Build history of the part. All positions in model axes, mm. A direction names the side the tool comes from. Round coordinates to 2 decimals unless told otherwise and drop trailing zeros. Loops run counter-clockwise (first coordinate to the right, second up) from the corner with the lowest first, then second, coordinate; pieces in that order, holes last. Notation, with made-up numbers: M 57,87 L 85,87 A16 cw 85,110 Z; hole C 41.25,71 d3. An arc over 180 degrees is marked long. One line per item, written item: value.
```python
from build123d import *

# Parameters (mm, degrees)
SKETCH1_W           = 85.598
SKETCH1_H           = 85.598
BOSS_EXTRUDE1_DEPTH = 66.04
CUT_EXTRUDE1_DEPTH  = 55.88
CUT_EXTRUDE2_DEPTH  = 55.88
CUT_EXTRUDE3_DEPTH  = 55.88
CUT_EXTRUDE4_DEPTH  = 55.88
CUT_EXTRUDE5_DEPTH  = 55.88
CUT_EXTRUDE6_DEPTH  = 55.88
CUT_EXTRUDE7_DEPTH  = 55.88
CUT_EXTRUDE8_DEPTH  = 55.88
SKETCH10_R          = 36.5125
BOSS_EXTRUDE2_DEPTH = 1.524
SKETCH11_R          = 6.35
BOSS_EXTRUDE3_DEPTH = 35.56
CUT_EXTRUDE9_DEPTH  = 25.4
CUT_EXTRUDE10_DEPTH = 25.4
SKETCH14_W          = 0.635
SKETCH14_H          = 71.501
SKETCH15_W          = 0.635
SKETCH15_H          = 71.501
SKETCH16_W          = 0.635
SKETCH16_H          = 71.501
SKETCH17_W          = 0.635
SKETCH17_H          = 71.501
HOLE1_D             = 6.604
HOLE1_DEPTH         = 47.244
HOLE2_D             = 6.604
HOLE2_DEPTH         = 47.244
HOLE3_D             = 6.604
HOLE3_DEPTH         = 47.244
HOLE4_D             = 6.604
HOLE4_DEPTH         = 47.244
CHAMFER1_SIZE       = 0.254
CHAMFER2_SIZE       = 0.254
FILLET1_R           = 2.54
FILLET2_R           = 2.54
FILLET3_R           = 2.54
FILLET4_R           = 2.54
FILLET5_R           = 2.54
FILLET6_R           = 2.54
FILLET7_R           = 2.54
FILLET8_R           = 2.54


with BuildPart() as part:
    # Sketch1 → Boss-Extrude1 (new body)
    with BuildSketch(Plane.XY.offset(66.04)):
        Rectangle(SKETCH1_W, SKETCH1_H)
    extrude(amount=-BOSS_EXTRUDE1_DEPTH)

    # Sketch2 → Cut-Extrude1 (cut)
    with BuildSketch(Plane(origin=(0, 0, 0), x_dir=(-1, 0, 0), z_dir=(0, 0, -1))):
        with BuildLine():
            Line((-42.799, -42.799), (-24.420683344, -42.799))
            ThreePointArc((-24.420683344, -42.799), (-34.84339375, -34.84339375), (-42.799, -24.420683344))
            Line((-42.799, -24.420683344), (-42.799, -42.799))
        make_face()
    extrude(amount=-CUT_EXTRUDE1_DEPTH, mode=Mode.SUBTRACT)

    # Sketch3 → Cut-Extrude2 (cut)
    with BuildSketch(Plane(origin=(0, 0, 0), x_dir=(-1, 0, 0), z_dir=(0, 0, -1))):
        with BuildLine():
            Line((-28.2194, -40.395416072), (-28.2194, -28.2194))
            Line((-28.2194, -28.2194), (-40.395416072, -28.2194))
            ThreePointArc((-40.395416072, -28.2194), (-34.84339375, -34.84339375), (-28.2194, -40.395416072))
        make_face()
    extrude(amount=-CUT_EXTRUDE2_DEPTH, mode=Mode.SUBTRACT)

    # Sketch4 → Cut-Extrude3 (cut)
    with BuildSketch(Plane(origin=(0, 0, 0), x_dir=(-1, 0, 0), z_dir=(0, 0, -1))):
        with BuildLine():
            Line((-42.799, 42.799), (-42.799, 24.420683344))
            ThreePointArc((-42.799, 24.420683344), (-34.84339375, 34.84339375), (-24.420683344, 42.799))
            Line((-24.420683344, 42.799), (-42.799, 42.799))
        make_face()
    extrude(amount=-CUT_EXTRUDE3_DEPTH, mode=Mode.SUBTRACT)

    # Sketch5 → Cut-Extrude4 (cut)
    with BuildSketch(Plane(origin=(0, 0, 0), x_dir=(-1, 0, 0), z_dir=(0, 0, -1))):
        with BuildLine():
            Line((-40.395416072, 28.2194), (-28.2194, 28.2194))
            Line((-28.2194, 28.2194), (-28.2194, 40.395416072))
            ThreePointArc((-28.2194, 40.395416072), (-34.84339375, 34.84339375), (-40.395416072, 28.2194))
        make_face()
    extrude(amount=-CUT_EXTRUDE4_DEPTH, mode=Mode.SUBTRACT)

    # Sketch6 → Cut-Extrude5 (cut)
    with BuildSketch(Plane(origin=(0, 0, 0), x_dir=(-1, 0, 0), z_dir=(0, 0, -1))):
        with BuildLine():
            Line((42.799, 42.799), (24.420683344, 42.799))
            ThreePointArc((24.420683344, 42.799), (34.84339375, 34.84339375), (42.799, 24.420683344))
            Line((42.799, 24.420683344), (42.799, 42.799))
        make_face()
    extrude(amount=-CUT_EXTRUDE5_DEPTH, mode=Mode.SUBTRACT)

    # Sketch7 → Cut-Extrude6 (cut)
    with BuildSketch(Plane(origin=(0, 0, 0), x_dir=(-1, 0, 0), z_dir=(0, 0, -1))):
        with BuildLine():
            Line((28.2194, 40.395416072), (28.2194, 28.2194))
            Line((28.2194, 28.2194), (40.395416072, 28.2194))
            ThreePointArc((40.395416072, 28.2194), (34.84339375, 34.84339375), (28.2194, 40.395416072))
        make_face()
    extrude(amount=-CUT_EXTRUDE6_DEPTH, mode=Mode.SUBTRACT)

    # Sketch8 → Cut-Extrude7 (cut)
    with BuildSketch(Plane(origin=(0, 0, 0), x_dir=(-1, 0, 0), z_dir=(0, 0, -1))):
        with BuildLine():
            Line((42.799, -42.799), (42.799, -24.420683344))
            ThreePointArc((42.799, -24.420683344), (34.84339375, -34.84339375), (24.420683344, -42.799))
            Line((24.420683344, -42.799), (42.799, -42.799))
        make_face()
    extrude(amount=-CUT_EXTRUDE7_DEPTH, mode=Mode.SUBTRACT)

    # Sketch9 → Cut-Extrude8 (cut)
    with BuildSketch(Plane(origin=(0, 0, 0), x_dir=(-1, 0, 0), z_dir=(0, 0, -1))):
        with BuildLine():
            Line((40.395416072, -28.2194), (28.2194, -28.2194))
            Line((28.2194, -28.2194), (28.2194, -40.395416072))
            ThreePointArc((28.2194, -40.395416072), (34.84339375, -34.84339375), (40.395416072, -28.2194))
        make_face()
    extrude(amount=-CUT_EXTRUDE8_DEPTH, mode=Mode.SUBTRACT)

    # Sketch10 → Boss-Extrude2 (add)
    with BuildSketch(Plane.XY.offset(66.04)):
        Circle(SKETCH10_R)
    extrude(amount=BOSS_EXTRUDE2_DEPTH)

    # Sketch11 → Boss-Extrude3 (add)
    with BuildSketch(Plane.XY.offset(67.564)):
        Circle(SKETCH11_R)
    extrude(amount=BOSS_EXTRUDE3_DEPTH)

    # Sketch12 → Cut-Extrude9 (cut)
    with BuildSketch(Plane.XY.offset(103.124)):
        with BuildLine():
            Line((-3.81, 5.08), (3.81, 5.08))
            ThreePointArc((3.81, 5.08), (0, 6.35), (-3.81, 5.08))
        make_face()
    extrude(amount=-CUT_EXTRUDE9_DEPTH, mode=Mode.SUBTRACT)

    # Sketch13 → Cut-Extrude10 (cut)
    with BuildSketch(Plane.XY.offset(103.124)):
        with BuildLine():
            Line((5.08, 3.81), (5.08, -3.81))
            ThreePointArc((5.08, -3.81), (6.35, 0), (5.08, 3.81))
        make_face()
    extrude(amount=-CUT_EXTRUDE10_DEPTH, mode=Mode.SUBTRACT)

    # Sketch14 → Revolve1 (revolve)
    with BuildSketch(Plane(origin=(0, 0, 12.7), x_dir=(-1, 0, 0), z_dir=(0, 0, -1))):
        with Locations((1.7145, 78.5495)):
            Rectangle(SKETCH14_W, SKETCH14_H)
    revolve(axis=Axis((-2.032, 42.799, 12.7), (0, 1, 0)))

    # Sketch15 → Revolve2 (revolve)
    with BuildSketch(Plane(origin=(0, 0, 12.7), x_dir=(-1, 0, 0), z_dir=(0, 0, -1))):
        with Locations((-2.3495, 78.5495)):
            Rectangle(SKETCH15_W, SKETCH15_H)
    revolve(axis=Axis((2.032, 42.799, 12.7), (0, 1, 0)))

    # Sketch16 → Revolve3 (revolve)
    with BuildSketch(Plane(origin=(0, 0, 14.732), x_dir=(-1, 0, 0), z_dir=(0, 0, -1))):
        with Locations((-0.3175, 78.5495)):
            Rectangle(SKETCH16_W, SKETCH16_H)
    revolve(axis=Axis((0, 42.799, 14.732), (0, 1, 0)))

    # Sketch17 → Revolve4 (revolve)
    with BuildSketch(Plane(origin=(0, 0, 10.668), x_dir=(-1, 0, 0), z_dir=(0, 0, -1))):
        with Locations((-0.3175, 78.5495)):
            Rectangle(SKETCH17_W, SKETCH17_H)
    revolve(axis=Axis((0, 42.799, 10.668), (0, 1, 0)))

    # Hole1
    with Locations(Plane(origin=(0, 0, 55.88), x_dir=(-1, 0, 0), z_dir=(0, 0, -1))):
        with Locations((34.798, -34.798)):
            Hole(HOLE1_D / 2, depth=HOLE1_DEPTH)

    # Hole2
    with Locations(Plane(origin=(0, 0, 55.88), x_dir=(-1, 0, 0), z_dir=(0, 0, -1))):
        with Locations((34.798, 34.798)):
            Hole(HOLE2_D / 2, depth=HOLE2_DEPTH)

    # Hole3
    with Locations(Plane(origin=(0, 0, 55.88), x_dir=(-1, 0, 0), z_dir=(0, 0, -1))):
        with Locations((-34.798, 34.798)):
            Hole(HOLE3_D / 2, depth=HOLE3_DEPTH)

    # Hole4
    with Locations(Plane(origin=(0, 0, 55.88), x_dir=(-1, 0, 0), z_dir=(0, 0, -1))):
        with Locations((-34.798, -34.798)):
            Hole(HOLE4_D / 2, depth=HOLE4_DEPTH)

    # Chamfer1
    chamfer1_edges = [part.edges().sort_by_distance(p)[0] for p in [
        (-4.490128061, -4.490128061, 103.124),
    ]]
    chamfer(chamfer1_edges, length=CHAMFER1_SIZE)

    # Chamfer2
    chamfer2_edges = [part.edges().sort_by_distance(p)[0] for p in [
        (4.490128061, 4.490128061, 103.124),
    ]]
    chamfer(chamfer2_edges, length=CHAMFER2_SIZE)

    # Fillet1
    fillet1_edges = [part.edges().sort_by_distance(p)[0] for p in [
        (-42.799, -42.799, 60.96),
    ]]
    fillet(fillet1_edges, radius=FILLET1_R)

    # Fillet2
    fillet2_edges = [part.edges().sort_by_distance(p)[0] for p in [
        (-42.799, 42.799, 60.96),
    ]]
    fillet(fillet2_edges, radius=FILLET2_R)

    # Fillet3
    fillet3_edges = [part.edges().sort_by_distance(p)[0] for p in [
        (42.799, 42.799, 60.96),
    ]]
    fillet(fillet3_edges, radius=FILLET3_R)

    # Fillet4
    fillet4_edges = [part.edges().sort_by_distance(p)[0] for p in [
        (-28.2194, 28.2194, 27.94),
    ]]
    fillet(fillet4_edges, radius=FILLET4_R)

    # Fillet5
    fillet5_edges = [part.edges().sort_by_distance(p)[0] for p in [
        (42.799, -42.799, 60.96),
    ]]
    fillet(fillet5_edges, radius=FILLET5_R)

    # Fillet6
    fillet6_edges = [part.edges().sort_by_distance(p)[0] for p in [
        (28.2194, -28.2194, 27.94),
    ]]
    fillet(fillet6_edges, radius=FILLET6_R)

    # Fillet7
    fillet7_edges = [part.edges().sort_by_distance(p)[0] for p in [
        (28.2194, 28.2194, 27.94),
    ]]
    fillet(fillet7_edges, radius=FILLET7_R)

    # Fillet8
    fillet8_edges = [part.edges().sort_by_distance(p)[0] for p in [
        (-28.2194, -28.2194, 27.94),
    ]]
    fillet(fillet8_edges, radius=FILLET8_R)


solid = part.part
```
Item 1: Slice it at D-D, the plane x = 21. Give the cut face in (y, z), and give its area (3 significant figures).
Check values:
outline: M -42.8,0 L 42.8,0 L 42.8,66.04 L 29.87,66.04 L 29.87,67.56 L -29.87,67.56 L -29.87,66.04 L -42.8,66.04 Z
area: 5,740 mm2
Item 2: Slice it at A-A, the plane x = 34. Give the cut face in (y, z).
Check values:
outline: M -42.8,55.88 L -38,55.88 L -38,66.04 L -42.8,66.04 Z; M -31.59,55.88 L -28.22,55.88 L -28.22,0 L 28.22,0 L 28.22,55.88 L 31.59,55.88 L 31.59,66.04 L 13.31,66.04 L 13.31,67.56 L -13.31,67.56 L -13.31,66.04 L -31.59,66.04 Z; M 38,55.88 L 42.8,55.88 L 42.8,66.04 L 38,66.04 Z
Item 3: Slice it at B-B, the plane z = 25. Give the cut face in (x, y).
Check values:
outline: M -42.8,-24.42 A49.28 ccw -40.4,-28.22 L -30.76,-28.22 A2.54 cw -28.22,-30.76 L -28.22,-40.4 A49.28 ccw -24.42,-42.8 L 24.42,-42.8 A49.28 ccw 28.22,-40.4 L 28.22,-30.76 A2.54 cw 30.76,-28.22 L 40.4,-28.22 A49.28 ccw 42.8,-24.42 L 42.8,24.42 A49.28 ccw 40.4,28.22 L 30.76,28.22 A2.54 cw 28.22,30.76 L 28.22,40.4 A49.28 ccw 24.42,42.8 L -24.42,42.8 A49.28 ccw -28.22,40.4 L -28.22,30.76 A2.54 cw -30.76,28.22 L -40.4,28.22 A49.28 ccw -42.8,24.42 Z
Item 4: Wall check: line 1 along Y through (x, z) = (-35.5, 59); line 2 along Y through (x, z) = (-1.5, 44); line 3 along Z through (x, y) = (30, -35). Give the ranges that are in metal, low to high.
Check values:
line 1: y = -42.8 to -38.02, -31.57 to 31.57, 38.02 to 42.8
line 2: y = -42.8 to 42.8
line 3: z = 55.88 to 66.04
Item 5: Pull direction Y, two halves, no side cores. Call faces 4 (the face through (-36, -28.219, 28)), 5 (the face through (38, -38, 55.88)), 6 (the face through (32.364, 37.03, 61.031)): pulls with the +Y half, pulls with the -Y half, needs draft (parallel to the pull), parting line crosses it, or undercut.
Check values:
face 4: pulls with the -Y half
face 5: needs draft
face 6: undercut
Item 6: Slice it at C-C, the plane y = 0. Give the cut face in (x, z).
Check values:
outline: M -42.8,0 L 42.8,0 L 42.8,66.04 L 36.51,66.04 L 36.51,67.56 L 6.35,67.56 L 6.35,77.72 L 5.08,77.72 L 5.08,103.12 L -6.1,103.12 L -6.35,102.87 L -6.35,67.56 L -36.51,67.56 L -36.51,66.04 L -42.8,66.04 Z
Item 7: Drop flat-ended pins along their axis: P1, Ø14.5, axis at x = 33, y = 32.5, coming from the -Z side; P2, Ø4, axis at x = -34.798, y = -34.798, coming from the -Z side; P3, Ø10, axis at x = -33.5, z = 11.5, coming from the -Y side; P4, Ø10, axis at y = 70.5, z = 15, coming from the -X side. Give the stop position or say it passes through.
Check values:
P1: stops at z = 0
P2: passes through
P3: stops at y = -29.6
P4: stops at x = -2.67
Item 8: Which spindle directions (+Z, -Z, +X, -X, +Y, -Y) get a long thin tool onto all of the face, cutting with end or side? Do faces 1 (the face through (41.66, 26.32, 27.55)), 2 (the face through (36, -28.219, 28)), 3 (the face through (5.08, 0, 91)). Say none if no direction does.
Check values:
face 1: -Z, +X, +Y
face 2: -Z, +X, -Y
face 3: +Z, +X, +Y, -Y
